from build123d import *

# Parameters (mm, degrees)
SKETCH1_R           = 28.1
BOSS_EXTRUDE2_DEPTH = 24
CUT_EXTRUDE2_DEPTH  = 21.5
SKETCH4_R           = 3
CUT_EXTRUDE3_DEPTH  = 9.5
SKETCH6_R           = 6.025
CUT_EXTRUDE4_DEPTH  = 6.2
SKETCH7_W           = 56.2
SKETCH7_H           = 56.2
BOSS_EXTRUDE3_DEPTH = 56.2
SKETCH8_W           = 56.2
SKETCH8_H           = 56.2
BOSS_EXTRUDE4_DEPTH = 14.14
SKETCH10_W          = 56.2
SKETCH10_H          = 56.2
BOSS_EXTRUDE5_DEPTH = 10
SKETCH19_W          = 51.2
SKETCH19_H          = 51.2
CUT_EXTRUDE5_DEPTH  = 63.7
SKETCH21_R          = 3
CUT_EXTRUDE7_DEPTH  = 20


with BuildPart() as part:
    # Sketch1 → Boss-Extrude2 (new body)
    with BuildSketch(Plane.XY):
        Circle(SKETCH1_R)
    extrude(amount=BOSS_EXTRUDE2_DEPTH)

    # Sketch3 → Cut-Extrude2 (cut)
    with BuildSketch(Plane(origin=(0, 0, 0), x_dir=(-1, 0, 0), z_dir=(0, 0, -1))):
        with BuildLine():
            Line((-1.661801922, 2.5), (1.661801922, 2.5))
            ThreePointArc((1.661801922, 2.5), (0, -3.001930317), (-1.661801922, 2.5))
        make_face()
    extrude(amount=-CUT_EXTRUDE2_DEPTH, mode=Mode.SUBTRACT)

    # Sketch4 → Cut-Extrude3 (cut)
    with BuildSketch(Plane(origin=(0, 0, 0), x_dir=(-1, 0, 0), z_dir=(0, 0, -1))):
        Circle(SKETCH4_R)
    extrude(amount=-CUT_EXTRUDE3_DEPTH, mode=Mode.SUBTRACT)

    # Sketch6 → Cut-Extrude4 (cut)
    with BuildSketch(Plane(origin=(0, 0, 0), x_dir=(-1, 0, 0), z_dir=(0, 0, -1))):
        Circle(SKETCH6_R)
    extrude(amount=-CUT_EXTRUDE4_DEPTH, mode=Mode.SUBTRACT)

    # Sketch7 → Boss-Extrude3 (add)
    with BuildSketch(Plane.XY.offset(24)):
        Rectangle(SKETCH7_W, SKETCH7_H)
    extrude(amount=BOSS_EXTRUDE3_DEPTH)

    # Sketch8 → Boss-Extrude4 (add)
    with BuildSketch(Plane(origin=(28.1, 0, 0), x_dir=(0, 0, -1), z_dir=(1, 0, 0))):
        with Locations((-52.1, 0)):
            Rectangle(SKETCH8_W, SKETCH8_H)
    extrude(amount=BOSS_EXTRUDE4_DEPTH)

    # Sketch10 → Boss-Extrude5 (add)
    with BuildSketch(Plane(origin=(42.24, 0, 0), x_dir=(0, 0, -1), z_dir=(1, 0, 0))):
        with Locations((-52.1, 0)):
            Rectangle(SKETCH10_W, SKETCH10_H)
    extrude(amount=BOSS_EXTRUDE5_DEPTH)

    # Sketch19 → Cut-Extrude5 (cut)
    with BuildSketch(Plane.ZY.offset(28.1)):
        with Locations((52.1, 0)):
            Rectangle(SKETCH19_W, SKETCH19_H)
    extrude(amount=-CUT_EXTRUDE5_DEPTH, mode=Mode.SUBTRACT)

    # Cut-Sweep2: sweep along a path in Sketch20
    with BuildLine(Plane(origin=(0, 0, 0), x_dir=(-1, 0, 0), z_dir=(0, 0, -1))) as cut_sweep2_path:
        ThreePointArc((0, 15), (-10.606601718, 10.606601718), (-15, 0))
    # 3DSketch2 → Cut-Sweep2 (sweep, cut)
    with BuildSketch(Plane(origin=(0, 15, 0), x_dir=(0, 0.17521220324553322, 0.9845306921746249), z_dir=(-1, 0, 0))):
        Polygon((0, 0), (1.314091524, 7.383980191), (42.805237655, 0), (41.491146131, -7.383980191), align=None)
    sweep(path=cut_sweep2_path.line, mode=Mode.SUBTRACT)

    # Sketch21 → Cut-Extrude7 (cut)
    with BuildSketch(Plane(origin=(52.24, 0, 0), x_dir=(0, 0, -1), z_dir=(1, 0, 0))):
        with Locations((-73.65, 21.55)):
            Circle(SKETCH21_R)
        with Locations((-30.55, 21.55)):
            Circle(SKETCH21_R)
        with Locations((-30.55, -21.55)):
            Circle(SKETCH21_R)
        with Locations((-73.65, -21.55)):
            Circle(SKETCH21_R)
    extrude(amount=-CUT_EXTRUDE7_DEPTH, mode=Mode.SUBTRACT)


solid = part.part
Here's how the part is built. I have some questions about the finished solid (model axes, mm). A direction names the side the tool comes from. Coordinates: 2 decimals unless noted, no trailing zeros. Order: outer loops, then holes, each group sorted by start corner. A loop starts at its lowest first (then second) coordinate and runs counter-clockwise, first axis right, second up.
Item 1: If we section it at B-B on x = 41.5: List the corners of the cut face in (y, z) for me.
Result sheet:
outline: (-28.1, 24) - (28.1, 24) - (28.1, 80.2) - (-28.1, 80.2) - close; hole circle Ø6 at (-21.55, 30.55); hole circle Ø6 at (-21.55, 73.65); hole circle Ø6 at (21.55, 30.55); hole circle Ø6 at (21.55, 73.65)
Item 2: If we section it at A-A on z = 73.65: List the corners of the cut face in (x, y) for me, plus the area to 3 significant figures.
Result sheet:
outline: (-28.1, -28.1) - (52.24, -28.1) - (52.24, -24.55) - (35.6, -24.55) - (35.6, -25.6) - (-28.1, -25.6) - close; (-28.1, 25.6) - (35.6, 25.6) - (35.6, 24.55) - (52.24, 24.55) - (52.24, 28.1) - (-28.1, 28.1) - close; (35.6, -18.55) - (52.24, -18.55) - (52.24, 18.55) - (35.6, 18.55) - close
area: 1,050 mm2
Item 3: For P1, Ø5, axis at y = 17.5, z = 14.5, coming from the +X side; P2, Ø6, axis at y = -11, z = 9.5, coming from the -X side; P3, Ø8, axis at y = -21.55, z = 73.65, coming from the -X side, each with a flat end and sliding along its axis, tell me the tip position at first contact or that it passes through.
Result sheet:
P1: stops at x = 23.76
P2: stops at x = -26.94
P3: stops at x = 35.6
Item 4: If we section it at D-D on y = 8: List the corners of the cut face in (x, z) for me, plus the area to 3 significant figures.
Result sheet:
outline: (-28.1, 24) - (-26.94, 24) - (-26.94, 0) - (12.69, 0) - (12.69, 26.5) - (-28.1, 26.5) - close; (-28.1, 77.7) - (35.6, 77.7) - (35.6, 26.5) - (21.03, 26.5) - (21.03, 0) - (26.94, 0) - (26.94, 24) - (52.24, 24) - (52.24, 80.2) - (-28.1, 80.2) - close
area: 2,330 mm2
Item 5: I need wall thicknesses on line 1 (Y direction, x = 26.5, z = 59); line 2 (Y direction, x = 46.5, z = 72); line 3 (Z direction, x = 15.5, y = -18.5). Which ranges of each line are inside material? Lowest first, please.
Result sheet:
line 1: y = -28.1 to -25.6, 25.6 to 28.1
line 2: y = -28.1 to -24.06, -19.04 to 19.04, 24.06 to 28.1
line 3: z = 0 to 26.5, 77.7 to 80.2
Item 6: If we section it at C-C on y = -16: List the corners of the cut face in (x, z) for me.
Result sheet:
outline: (-28.1, 24) - (-23.1, 24) - (-23.1, 0) - (23.1, 0) - (23.1, 24) - (52.24, 24) - (52.24, 80.2) - (-28.1, 80.2) - (-28.1, 77.7) - (35.6, 77.7) - (35.6, 26.5) - (-28.1, 26.5) - close
Item 7: For faces 1 (the face through (3, 0, 77.7)), 2 (the face through (-22, -21, 24)), 3 (the face through (0, 19, 13)), which set-ups out of +Z, -Z, +X, -X, +Y, -Y let a thin tool reach every point of the face, with its end or its side?
Result sheet:
face 1: -X
face 2: -Z, -X, -Y
face 3: -Z
Item 8: If we mould it in two halves opening along X, with no side actions, what happens to faces 4 (the face through (44.04, 22.45, 70.79)), 5 (the face through (35.6, 0, 52)), 6 (the face through (0, -3, 14)), 7 (the face through (-6.092, -27.432, 11.832))? For each: +X half, -X half, draft (parallel to the pull), parting line (faces both ways), or undercut.
Result sheet:
face 4: draft
face 5: -X half
face 6: undercut
face 7: parting line
